Input: part model. Units: mm. Frame: model coordinates. Face numbers are marked on the shaded views. A direction names the side the tool comes from. Round coordinates to 2 decimals unless told otherwise and drop trailing zeros. Loops run counter-clockwise (first coordinate to the right, second up) from the corner with the lowest first, then second, coordinate; pieces in that order, holes last. Notation, with made-up numbers: (-36, 49) -> (-15, 49) arc R21 ccw to (-15, 58) -> close; hole circle Ø5 at (71.25, 53). An arc over 180 degrees is marked (long way). Answer as a JSON object with one key per item and string values. Group by question number.
Item 1: Material intervals for line 1 (Z direction, x = 48.5, y = 13.25); line 2 (Y direction, x = -7, z = 7.5); line 3 (Y direction, x = 65.5, z = 3), sorted ascending. Write a range as [from, to].
Item 2: Section query A-A on x = 85.5. Return loops of the section in (y, z).
Item 3: Pin query (flat end, axial travel): pin 1 (8 mm diameter, centred on x = 2, z = 7, fed in from +Y); pin 2 (16.5 mm diameter, centred on x = -10, y = 23.5, fed in from +Z); pin 3 (10.5 mm diameter, centred on x = -4.5, z = 16, fed in from +Y). Return the tip coordinate at first contact, or that it passes through.
Item 4: Section query C-C on y = 14.25. Return loops of the section in (x, z).
Item 5: Section query B-B on z = 16. Return loops of the section in (x, y), and give its area (3 significant figures).
Item 6: Set-up query: the marked faces 1 and 2. Return all of +Z, -Z, +X, -X, +Y, -Y with unobstructed straight access to the full face (end or side cutting, diameter ignored); none if empty.
Item 7: Section query D-D on x = -17. Return loops of the section in (y, z), and give its area (3 significant figures).
from build123d import *

# Parameters (mm, degrees)
EXTRUDE_1_DEPTH     = 104
CUT_EXTRUDE_1_DEPTH = 113.320968657


with BuildPart() as part:
    # Эскиз1 → Бобышка-Вытянуть1 (new, symmetric)
    with BuildSketch(Plane(origin=(0, 0, 0), x_dir=(0, 0, -1), z_dir=(1, 0, 0))):
        with BuildLine():
            Line((0, 0), (0, 30))
            Line((0, 30), (-2.7, 30))
            ThreePointArc((-2.7, 30), (-3.619238816, 29.619238816), (-4, 28.7))
            Line((-4, 28.7), (-4, 8))
            ThreePointArc((-4, 8), (-5.171572875, 5.171572875), (-8, 4))
            Line((-8, 4), (-28.7, 4))
            ThreePointArc((-28.7, 4), (-29.619238816, 3.619238816), (-30, 2.7))
            Line((-30, 2.7), (-30, 0))
            Line((-30, 0), (0, 0))
        make_face()
    extrude(amount=EXTRUDE_1_DEPTH, both=True)

    # Эскиз2 → Вырез-Вытянуть1 (cut, through all)
    with BuildSketch(Plane.XZ):
        Polygon((-104, 4), (-78, 30), (-104, 30), align=None)
        Polygon((104, 4), (78, 30), (104, 30), align=None)
    extrude(amount=-CUT_EXTRUDE_1_DEPTH, mode=Mode.SUBTRACT)


solid = part.part
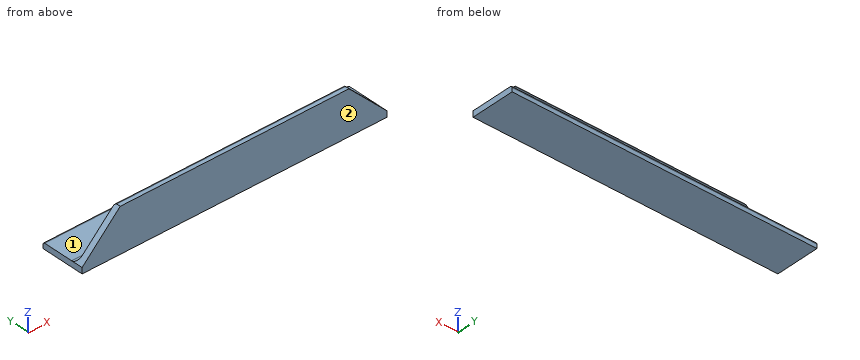
Solved:
{
 "1": {"line 1": "[0, 4]", "line 2": "[0, 4.03]", "line 3": "[0, 29.96]"},
 "2": {"outline": "(0, 0) -> (30, 0) -> (30, 2.7) arc R1.3 ccw to (28.7, 4) -> (8, 4) arc R4 cw to (4, 8) -> (4, 22.5) -> (0, 22.5) -> close"},
 "3": {"pin 1": "y = 29.96", "pin 2": "z = 4", "pin 3": "y = 4"},
 "4": {"outline": "(-104, 0) -> (104, 0) -> (104, 4) -> (-104, 4) -> close"},
 "5": {"outline": "(-92, 0) -> (92, 0) -> (92, 4) -> (-92, 4) -> close", "area": "736 mm²"},
 "6": {"face 1": "+Z, +X, -X, +Y", "face 2": "+Z, -Z, +X, -X, -Y"},
 "7": {"outline": "(0, 0) -> (30, 0) -> (30, 2.7) arc R1.3 ccw to (28.7, 4) -> (8, 4) arc R4 cw to (4, 8) -> (4, 28.7) arc R1.3 ccw to (2.7, 30) -> (0, 30) -> close", "area": "227 mm²"}
}
